from build123d import *

# Parameters (mm, degrees)
SKETCH3_W           = 0.64
SKETCH3_H           = 0.64
BOSS_EXTRUDE1_DEPTH = 5


with BuildPart() as part:
    # Sketch2 → Base-Revolve (revolve)
    with BuildSketch(Plane(origin=(0, 0, 0), x_dir=(0, 0, -1), z_dir=(1, 0, 0))):
        with BuildLine():
            Line((0, 0), (0, 2.55))
            Line((0, 2.55), (-1, 2.55))
            Line((-1, 2.55), (-1, 2.05))
            Line((-1, 2.05), (-6.55, 2.05))
            ThreePointArc((-6.55, 2.05), (-7.999568901, 1.449568901), (-8.6, 0))
            Line((-8.6, 0), (0, 0))
        make_face()
    revolve(axis=Axis((0, 0, 0), (0, 0, 1)))

    # Sketch3 → Boss-Extrude1 (add)
    with BuildSketch(Plane(origin=(0, 0, 0), x_dir=(-1, 0, 0), z_dir=(0, 0, -1))):
        with Locations((0, 1.27)):
            Rectangle(SKETCH3_W, SKETCH3_H)
        with Locations((0, -1.27)):
            Rectangle(SKETCH3_W, SKETCH3_H)
    extrude(amount=BOSS_EXTRUDE1_DEPTH)


solid = part.part
Build history of the part. All positions in model axes, mm. A direction names the side the tool comes from. Give positions to 0.01 mm unless a question says otherwise; leave off trailing zeros. Order: outer loops, then holes, each group sorted by start corner. A loop starts at its lowest first (then second) coordinate and runs counter-clockwise, first axis right, second up. Notation, with made-up numbers: M -34,-12 L 4,-12 A5 ccw 4,-3 Z; hole C 69.25,-23 d6. An arc over 180 degrees is marked long. Use one line per item in the form item = value.
Q1. Which spindle directions (+Z, -Z, +X, -X, +Y, -Y) get a long thin tool onto all of the face, cutting with end or side? Do faces 1 (the cylindrical face through (-2.033, -0.267, 3.814)), 2 (the cylindrical face through (2.26, 1.18, 0.51)). Say none if no direction does.
Conclusion:
face_1 = +Z
face_2 = +Z, -Z
Q2. Slice it at C-C, the plane z = 3. Write the cut outline in (x, y).
Conclusion:
outline = C 0,0 d4.1
Q3. Slice it at A-A, the plane x = 0. Write the cut outline in (y, z).
Conclusion:
outline = M -2.55,0 L -1.59,0 L -1.59,-5 L -0.95,-5 L -0.95,0 L 0.95,0 L 0.95,-5 L 1.59,-5 L 1.59,0 L 2.55,0 L 2.55,1 L 2.05,1 L 2.05,6.55 A2.05 ccw -2.05,6.55 L -2.05,1 L -2.55,1 Z
Q4. Pin check, flat tips, straight feed: P1, Ø2, axis at y = 0, z = 6, coming from the +X side; P2, Ø0.7, axis at y = 1, z = -2.5, coming from the +X side; P3, Ø0.5, axis at x = 0, z = -1.5, coming from the -Y side. Stop position of each tip, or through.
Conclusion:
P1 = 2.05
P2 = 0.32
P3 = -1.59
Q5. Wall check: probe 1 along Y at (x, z) = (-0.05, 5.75); probe 2 along Z at (x, y) = (1, -1.85); probe 3 along Y at (x, z) = (0.8, 0.5). Give the ranges that are in metal, low to high.
Conclusion:
probe_1 = -2.05 to 2.05
probe_2 = 0 to 1
probe_3 = -2.42 to 2.42
Q6. Slice it at D-D, the plane x = 1.85. Write the cut outline in (y, z) (3 decimals).
Conclusion:
outline = M -1.755,0 L 1.755,0 L 1.755,1 L 0.883,1 L 0.883,6.55 A0.883 ccw -0.883,6.55 L -0.883,1 L -1.755,1 Z
Q7. Slice it at B-B, the plane y = 0. Write the cut outline in (x, z).
Conclusion:
outline = M -2.55,0 L 2.55,0 L 2.55,1 L 2.05,1 L 2.05,6.55 A2.05 ccw -2.05,6.55 L -2.05,1 L -2.55,1 Z
